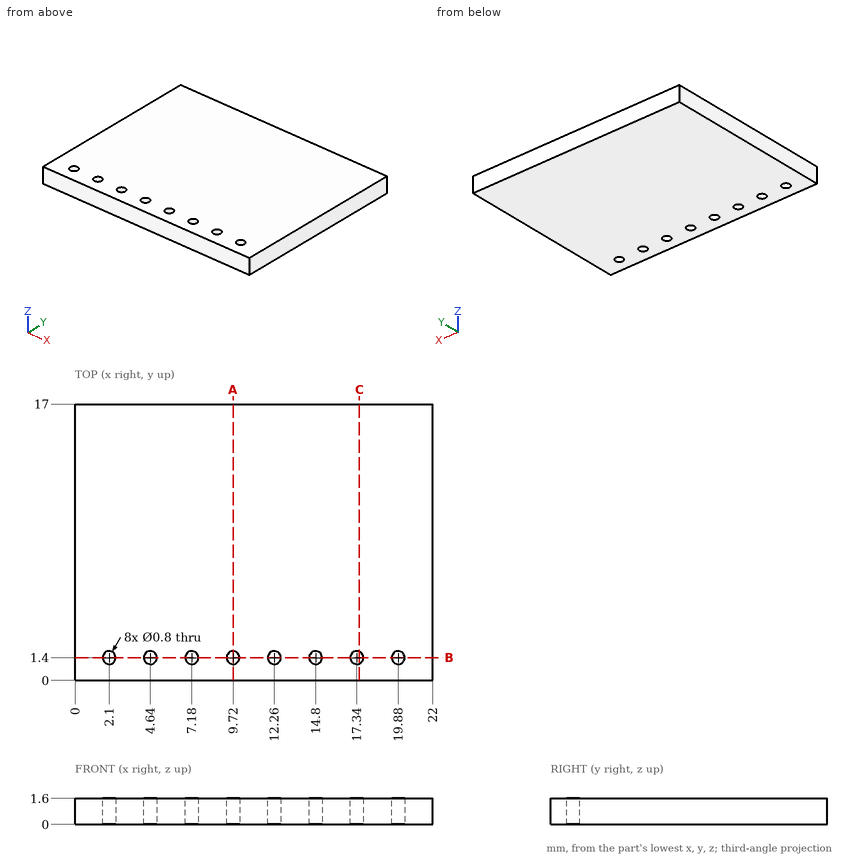
Geometry check sheet. Reference: drawing and pictorial views, mm from the part's lowest x, y, z. Round coordinates to 2 decimals unless told otherwise and drop trailing zeros. Order: outer loops, then holes, each group sorted by start corner. A loop starts at its lowest first (then second) coordinate and runs counter-clockwise, first axis right, second up.
Q1. Cross-section at C-C, the plane x = 17.5. Enter the section's corners in (y, z).
Filled sheet:
outline: (0, 0) - (1.03, 0) - (1.03, 1.6) - (0, 1.6) - close; (1.77, 0) - (17, 0) - (17, 1.6) - (1.77, 1.6) - close
Q2. Depth check by flat-ended pin: P1, Ø5, axis at x = 19, y = 13.5, coming from the -Z side. Enter the tip coordinate at first touch or a pass-through.
Filled sheet:
P1: stops at z = 0
Q3. Cross-section at B-B, the plane y = 1.4. Give the number of separate pieces and of enclosed holes in the cut face, plus the area to 3 significant figures.
Filled sheet:
separate pieces: 9
enclosed holes: 0
area: 25.0 mm2
Q4. Cross-section at A-A, the plane x = 9.72. Enter the section's corners in (y, z), plus the area to 3 significant figures.
Filled sheet:
outline: (0, 0) - (1, 0) - (1, 1.6) - (0, 1.6) - close; (1.8, 0) - (17, 0) - (17, 1.6) - (1.8, 1.6) - close
area: 25.9 mm2
Q5. Scan lines: L1, parallel to Y at x = 7.18, z = 1.15; L2, parallel to Y at x = 14.5, z = 1.4. Record each from-to range of solid material in increasing order.
Filled sheet:
L1: y = 0 to 1, 1.8 to 17
L2: y = 0 to 1.14, 1.66 to 17
